```python
from build123d import *

# Parameters (mm, degrees)
SKETCH_1_W                = 29
SKETCH_1_H                = 29
EXTRUDE_1_DEPTH           = 5
SKETCH_2_W                = 25
SKETCH_2_H                = 25
CUT_EXTRUDE_1_DEPTH       = 3
SKETCH_3_W                = 35
SKETCH_3_H                = 29
EXTRUDE_747_DEPTH         = 25.341167732
HOLE_WIZARD_M4_1_D        = 3.3
HOLE_WIZARD_M4_1_DEPTH    = 10.1
HOLE_WIZARD_M4_1_TIP      = 0.991420021
SKETCH_9_R                = 1
CUT_EXTRUDE_2_DEPTH       = 3
SKETCH_11_W               = 29
SKETCH_11_H               = 5
EXTRUDE_4_DEPTH           = 6
CUT_EXTRUDE_8_DEPTH       = 40.383835
SKETCH_19_W               = 80
SKETCH_19_H               = 25
EXTRUDE_5_DEPTH           = 10
HOLE_WIZARD_1_D           = 6.6
HOLE_WIZARD_1_DEPTH       = 10.1
HOLE_WIZARD_1_CBORE_D     = 11
HOLE_WIZARD_1_CBORE_DEPTH = 6.8
HOLE_WIZARD_1_TIP         = 1.982840043
SKETCH_23_W               = 80
SKETCH_23_H               = 10
EXTRUDE_6_DEPTH           = 2
SKETCH_24_W               = 27
SKETCH_24_H               = 10
CUT_EXTRUDE_9_DEPTH       = 2
MM_1_D                    = 4
MM_1_DEPTH                = 5
MM_1_TIP                  = 1.201721238
CUT_EXTRUDE_10_DEPTH      = 5
SKETCH_28_R               = 1
CUT_EXTRUDE_11_DEPTH      = 2
HOLE_WIZARD_M6_1_D        = 5
HOLE_WIZARD_M6_1_DEPTH    = 10
HOLE_WIZARD_M6_1_TIP      = 1.502151548
CUT_EXTRUDE_12_DEPTH      = 62.837260656
CUT_EXTRUDE_12_DEPTH_BACK = 62.837260656
SKETCH_32_W               = 27
SKETCH_32_H               = 10
CUT_EXTRUDE_13_DEPTH      = 6.5
SKETCH_33_W               = 27
SKETCH_33_H               = 10
CUT_EXTRUDE_14_DEPTH      = 6.5
CUT_EXTRUDE_15_DEPTH      = 5
MM_2_D                    = 4
MM_2_DEPTH                = 5
MM_2_TIP                  = 1.201721238
MM_3_D                    = 4
MM_3_DEPTH                = 5
MM_3_TIP                  = 1.201721238
SKETCH_38_W               = 23.961905905
SKETCH_38_H               = 13.839319444
EXTRUDE_7_DEPTH           = 27


with BuildPart() as part:
    # 草图1 → 凸台-拉伸1 (new body)
    with BuildSketch(Plane(origin=(0, 0, 0), x_dir=(1, 0, 0), z_dir=(0, 1, 0))):
        Rectangle(SKETCH_1_W, SKETCH_1_H)
    extrude(amount=EXTRUDE_1_DEPTH)

    # 草图2 → 切除-拉伸1 (cut)
    with BuildSketch(Plane.XZ.offset(-5)):
        Rectangle(SKETCH_2_W, SKETCH_2_H)
    extrude(amount=CUT_EXTRUDE_1_DEPTH, mode=Mode.SUBTRACT)

    # 草图3 → Extrude 747 (add)
    with BuildSketch(Plane(origin=(0, 0, 0), x_dir=(-1, 0, 0), z_dir=(0, -1, 0))):
        with Locations((3, 0)):
            Rectangle(SKETCH_3_W, SKETCH_3_H)
    extrude(amount=EXTRUDE_747_DEPTH)

    # M4 螺纹孔1
    with Locations(Plane.ZX.offset(2)):
        with Locations((0, 0)):
            Hole(HOLE_WIZARD_M4_1_D / 2, depth=HOLE_WIZARD_M4_1_DEPTH)
            with Locations((0, 0, -(HOLE_WIZARD_M4_1_DEPTH + HOLE_WIZARD_M4_1_TIP / 2))):  # 118° drill point
                Cone(0, HOLE_WIZARD_M4_1_D / 2, HOLE_WIZARD_M4_1_TIP, mode=Mode.SUBTRACT)

    # 草图9 → 切除-拉伸2 (cut)
    with BuildSketch(Plane(origin=(0, 5, 0), x_dir=(1, 0, 0), z_dir=(0, 1, 0))):
        with Locations((-12.5, 12.5)):
            Circle(SKETCH_9_R)
    extrude(amount=-CUT_EXTRUDE_2_DEPTH, mode=Mode.SUBTRACT)

    # 草图11 → 凸台-拉伸4 (add)
    with BuildSketch(Plane.ZY.offset(14.5)):
        with Locations((0, 2.5)):
            Rectangle(SKETCH_11_W, SKETCH_11_H)
    extrude(amount=EXTRUDE_4_DEPTH)

    # 草图17 → 切除-拉伸8 (cut, through all)
    with BuildSketch(Plane(origin=(0, 5, 0), x_dir=(1, 0, 0), z_dir=(0, 1, 0))):
        Polygon((-20.5, -14.5), (14.5, -14.5), (14.5, 14.5), (12.5, 14.5), (12.5, -12.5), (-20.5, -12.5), align=None)
    extrude(amount=-CUT_EXTRUDE_8_DEPTH, mode=Mode.SUBTRACT)

    # 草图19 → 凸台-拉伸5 (add)
    with BuildSketch(Plane(origin=(0, -25.341167732, 0), x_dir=(-1, 0, 0), z_dir=(0, -1, 0))):
        with Locations((6, 0)):
            Rectangle(SKETCH_19_W, SKETCH_19_H)
    extrude(amount=-EXTRUDE_5_DEPTH)

    # 打孔尺寸(%根据)内六角圆柱头螺钉的类型1
    with Locations(Plane(origin=(-31, -15.341167732, 0), x_dir=(0, 0, 1), z_dir=(0, 1, 0))):
        with Locations((0, 0), (0, 50)):
            CounterBoreHole(HOLE_WIZARD_1_D / 2, HOLE_WIZARD_1_CBORE_D / 2, HOLE_WIZARD_1_CBORE_DEPTH, depth=HOLE_WIZARD_1_DEPTH)
            with Locations((0, 0, -(HOLE_WIZARD_1_DEPTH + HOLE_WIZARD_1_TIP / 2))):  # 118° drill point
                Cone(0, HOLE_WIZARD_1_D / 2, HOLE_WIZARD_1_TIP, mode=Mode.SUBTRACT)

    # 草图23 → 凸台-拉伸6 (add)
    with BuildSketch(Plane(origin=(0, 0, -12.5), x_dir=(-1, 0, 0), z_dir=(0, 0, -1))):
        with Locations((6, -20.341167732)):
            Rectangle(SKETCH_23_W, SKETCH_23_H)
    extrude(amount=EXTRUDE_6_DEPTH)

    # 草图24 → 切除-拉伸9 (cut)
    with BuildSketch(Plane.ZY.offset(46)):
        with Locations((-1, -20.341167732)):
            Rectangle(SKETCH_24_W, SKETCH_24_H)
    extrude(amount=-CUT_EXTRUDE_9_DEPTH, mode=Mode.SUBTRACT)

    # 大小mm 暗销孔1
    with Locations(Plane(origin=(-21, -25.341167732, 0), x_dir=(0, 0, -1), z_dir=(0, -1, 0))):
        with Locations((0, 0)):
            Hole(MM_1_D / 2, depth=MM_1_DEPTH)
            with Locations((0, 0, -(MM_1_DEPTH + MM_1_TIP / 2))):  # 118° drill point
                Cone(0, MM_1_D / 2, MM_1_TIP, mode=Mode.SUBTRACT)

    # 草图27 → 切除-拉伸10 (cut)
    with BuildSketch(Plane.XZ.offset(25.341167732)):
        with BuildLine():
            Line((8.5, 2), (9.5, 2))
            ThreePointArc((9.5, 2), (11.5, 0), (9.5, -2))
            Line((9.5, -2), (8.5, -2))
            ThreePointArc((8.5, -2), (6.5, 0), (8.5, 2))
        make_face()
    extrude(amount=-CUT_EXTRUDE_10_DEPTH, mode=Mode.SUBTRACT)

    # 草图28 → 切除-拉伸11 (cut)
    with BuildSketch(Plane.XY.offset(12.5)):
        with Locations((-6, -5.341167732)):
            Circle(SKETCH_28_R)
    extrude(amount=-CUT_EXTRUDE_11_DEPTH, mode=Mode.SUBTRACT)

    # M6 螺纹孔1
    with Locations(Plane(origin=(-6, -25.341167732, 0), x_dir=(0, 0, -1), z_dir=(0, -1, 0))):
        with Locations((0, 0)):
            Hole(HOLE_WIZARD_M6_1_D / 2, depth=HOLE_WIZARD_M6_1_DEPTH)
            with Locations((0, 0, -(HOLE_WIZARD_M6_1_DEPTH + HOLE_WIZARD_M6_1_TIP / 2))):  # 118° drill point
                Cone(0, HOLE_WIZARD_M6_1_D / 2, HOLE_WIZARD_M6_1_TIP, mode=Mode.SUBTRACT)

    # 草图31 → 切除-拉伸12 (cut, two sides: drawn at the far end of the back side and taken through both)
    with BuildSketch(Plane(origin=(-6.0032, 14.658832268, 10.4718), x_dir=(1, 0, 0), z_dir=(0, 0, 1)).offset(-CUT_EXTRUDE_12_DEPTH_BACK)):
        with BuildLine():
            Line((10.117055245, -31.7), (8.854085532, -31.7))
            Line((8.854085532, -31.7), (6.07517942, -36.564132504))
            Line((6.07517942, -36.564132504), (6.531795149, -36.824999624))
            Line((6.531795149, -36.824999624), (10.275, -36.824999624))
            ThreePointArc((10.275, -36.824999624), (11.025, -37.574999624), (10.275, -38.324999624))
            Line((10.275, -38.324999624), (9.525, -38.324999624))
            Line((9.525, -38.324999624), (9.525, -40))
            Line((9.525, -40), (-9.776101272, -40))
            Line((-9.776101272, -40), (-9.776101272, -38.074384714))
            Line((-9.776101272, -38.074384714), (-10.526101272, -38.074384714))
            ThreePointArc((-10.526101272, -38.074384714), (-11.276101272, -37.324384714), (-10.526101272, -36.574384714))
            Line((-10.526101272, -36.574384714), (-6.501264425, -36.574384714))
            Line((-6.501264425, -36.574384714), (-6.501264425, -36.324384714))
            Line((-6.501264425, -36.324384714), (-9.143201284, -31.7))
            Line((-9.143201284, -31.7), (-10.369175052, -31.7))
            ThreePointArc((-10.369175052, -31.7), (-11.119175052, -30.95), (-10.369175052, -30.2))
            Line((-10.369175052, -30.2), (10.117055245, -30.2))
            ThreePointArc((10.117055245, -30.2), (10.867055245, -30.95), (10.117055245, -31.7))
        make_face()
    extrude(amount=CUT_EXTRUDE_12_DEPTH + CUT_EXTRUDE_12_DEPTH_BACK, mode=Mode.SUBTRACT)

    # 草图32 → 切除-拉伸13 (cut)
    with BuildSketch(Plane.ZY.offset(44)):
        with Locations((-1, -20.341167732)):
            Rectangle(SKETCH_32_W, SKETCH_32_H)
    extrude(amount=-CUT_EXTRUDE_13_DEPTH, mode=Mode.SUBTRACT)

    # 草图33 → 切除-拉伸14 (cut)
    with BuildSketch(Plane(origin=(34, 0, 0), x_dir=(0, 0, -1), z_dir=(1, 0, 0))):
        with Locations((1, -20.341167732)):
            Rectangle(SKETCH_33_W, SKETCH_33_H)
    extrude(amount=-CUT_EXTRUDE_14_DEPTH, mode=Mode.SUBTRACT)

    # 草图35 → 切除-拉伸15 (cut)
    with BuildSketch(Plane.XZ.offset(25.341167732)):
        with BuildLine():
            Line((8.5, -6), (9.5, -6))
            ThreePointArc((9.5, -6), (11.5, -8), (9.5, -10))
            Line((9.5, -10), (8.5, -10))
            ThreePointArc((8.5, -10), (6.5, -8), (8.5, -6))
        make_face()
    extrude(amount=-CUT_EXTRUDE_15_DEPTH, mode=Mode.SUBTRACT)

    # 大小mm 暗销孔2
    with Locations(Plane(origin=(-21, -25.341167732, -8), x_dir=(0, 0, -1), z_dir=(0, -1, 0))):
        with Locations((0, 0)):
            Hole(MM_2_D / 2, depth=MM_2_DEPTH)
            with Locations((0, 0, -(MM_2_DEPTH + MM_2_TIP / 2))):  # 118° drill point
                Cone(0, MM_2_D / 2, MM_2_TIP, mode=Mode.SUBTRACT)

    # 大小mm 暗销孔3
    with Locations(Plane(origin=(-21, -25.341167732, 8), x_dir=(0, 0, -1), z_dir=(0, -1, 0))):
        with Locations((0, 0)):
            Hole(MM_3_D / 2, depth=MM_3_DEPTH)
            with Locations((0, 0, -(MM_3_DEPTH + MM_3_TIP / 2))):  # 118° drill point
                Cone(0, MM_3_D / 2, MM_3_TIP, mode=Mode.SUBTRACT)

    # 草图38 → 凸台-拉伸7 (add)
    with BuildSketch(Plane.XY.offset(12.5)):
        with Locations((-6.428193068, -18.42150801)):
            Rectangle(SKETCH_38_W, SKETCH_38_H)
    extrude(amount=-EXTRUDE_7_DEPTH)


solid = part.part
```
The listing builds one solid part. Answer for the finished solid, in the listing's coordinates (mm). A direction names the side the tool comes from. Give positions to 0.01 mm unless a question says otherwise; leave off trailing zeros. Loops run counter-clockwise (first coordinate to the right, second up) from the corner with the lowest first, then second, coordinate; pieces in that order, holes last. Notation, with made-up numbers: (43.25, -31) - (76.25, -31) arc R25 cw to (76.25, -12) - close; hole circle Ø2 at (26.25, -37.5). An arc over 180 degrees is marked (long way). Return JSON: item names as keys, results as strings. Group by question number.
1. Given pin 1 Ø6 at (y, z) = (-1.5, 4) entering from -X; pin 2 Ø6 at (y, z) = (-1, 7) entering from +X; pin 3 Ø1.6 at (x, y) = (-6, -5.34) entering from +Z, each flat-ended and moving along its own axis, determine where each tip first touches the part or whether it passes through.
2. Find section C-C (y = -11.5). Write down the section's boundary in (x, z).
3. Determine the mould class of faces 1 (the cylindrical face through (-19, -23, 0)), 2 (the flat face through (23, -15.341, -4)), 3 (the flat face through (27.5, -20, -1)) for opening direction X: pulls with the +X half, pulls with the -X half, needs draft (parallel to the pull), parting line crosses it, or undercut.
4. Straight lines are drawn through the part: line 1 (Z direction, x = -21, y = -22.55); line 2 (X direction, y = -21.4, z = 0); line 3 (Z direction, x = 0, y = -3). For each, find the intervals that lie inside material, in ascending order. Write a range as [from, to].
5. Find section D-D (z = -0.75). State how many separate pieces and enclosed holes the cut face has, then the cut area to 4 significant figures.
6. Which of the six approach directions +Z, -Z, +X, -X, +Y, -Y give full straight-line access (tool end or side, diameter ignored) to faces 4 (the flat face through (-27, -15.341, -4)), 5 (the cylindrical face through (24.453, -18.694, -0.716)), 6 (the flat face through (12.5, -5, -1)), 7 (the cylindrical face through (-19, -23, 8))?
7. Find section B-B (y = -2.5). Write down the section's boundary in (x, z), then the cut area to 3 significant figures.
8. Find section A-A (x = 19). Write down the section's boundary in (y, z), then the cut area to 3 significant figures.
Verdict:
{
 "1": {"pin 1": "stops at x = -20.5", "pin 2": "stops at x = 12.5", "pin 3": "stops at z = 10.5"},
 "2": {"outline": "(-20.5, -14.5) - (12.5, -14.5) - (12.5, 12.5) - (-20.5, 12.5) - close"},
 "3": {"face 1": "undercut", "face 2": "needs draft", "face 3": "pulls with the +X half"},
 "4": {"line 1": "z = [-14.5, -10], [-6, -2], [2, 6], [10, 12.5]", "line 2": "x = [-37.5, -36.5], [-25.5, -23], [-19, 6.5], [11.5, 13.5], [24.5, 27.5]", "line 3": "z = [-14.5, -1.65], [1.65, 12.5]"},
 "5": {"separate pieces": "3", "enclosed holes": "0", "area": "982.5 mm^2"},
 "6": {"face 4": "+Z, -Z, -X, +Y", "face 5": "+Y", "face 6": "+Z, -Z, +X, +Y", "face 7": "-Y"},
 "7": {"outline": "(-20.5, -14.5) - (12.5, -14.5) - (12.5, 12.5) - (-20.5, 12.5) - close; hole circle Ø3.3 at (0, 0)", "area": "882 mm^2"},
 "8": {"outline": "(-25.34, -14.5) - (-15.34, -14.5) - (-15.34, -5.5) - (-22.14, -5.5) - (-22.14, -3.3) - (-25.34, -3.3) - close; (-25.34, 3.3) - (-22.14, 3.3) - (-22.14, 5.5) - (-15.34, 5.5) - (-15.34, 12.5) - (-25.34, 12.5) - close", "area": "174 mm^2"}
}
